Design review of the part built by this model. Coordinates are the model's own, in mm. A direction names the side the tool comes from. Round coordinates to 2 decimals unless told otherwise and drop trailing zeros. Write each loop counter-clockwise with the first axis right and the second up, starting at its lowest first coordinate (ties: lowest second). Pieces come first, ordered by that corner, then holes. Notation, with made-up numbers: (20.25, -19) -> (64.25, -19) arc R34 cw to (64.25, 16) -> close; hole circle Ø8 at (28.5, 87.5). An arc over 180 degrees is marked (long way). Write item = value, one per line. Start each with the question number.
Item 1: Add section C-C, the plane y = -11. State the section outline as (x, z) points.
Item 2: Machinability: for faces 1 (the flat face through (32, -20, 82)), 2 (the cylindrical face through (-304.222, -44.93, 73.268)), 3 (the flat face through (348.597, -20, 28)), which of the approach directions +Z, -Z, +X, -X, +Y, -Y give a long, thin tool a straight path to every point of the face, cutting with its end or side? Answer none if there is none.
Item 3: Add section B-B, the plane z = 125.5. State the section outline as (x, y) points, then the cut area to 3 significant figures.
Item 4: To check wall thickness, follow L1, parallel to Z at x = -25, y = -16.5; L2, parallel to Z at x = 13, y = -36; L3, parallel to X at y = -24, z = 125. State the ranges of each line that lie inside material, in increasing order.
Item 5: Add section D-D, the plane x = -129. State the section outline as (y, z) points.
Item 6: Add section A-A, the plane x = 25. State the section outline as (y, z) points.
Item 7: Mouldability with a two-part tool opening along Z and no side actions: class faces 4 (the cylindrical face through (-27.71, -19.72, 174.59)), 5 (the flat face through (-311, -50, 103)), 6 (the cylindrical face through (-290.5, -44.9, 75.8)) as released by +Z, released by -Z, zero draft, split by the parting line, or undercut.
from build123d import *

# Parameters (mm, degrees)
F1_W     = 560
F1_H     = 350
F1_W_2   = 111
F1_H_2   = 65
F1_R     = 68
F1_R_2   = 12.5
F1_W_3   = 64
F1_H_3   = 124
F1_W_4   = 30
F1_H_4   = 14
F1_R_3   = 11
F2_DEPTH = 40
F1_W_5   = 70
F3_DEPTH = 40
F4_DEPTH = 270
F6_DEPTH = 10


with BuildPart() as f2:
    # F1 (on Front) → F2 (new body)
    with BuildSketch(Plane.XZ):
        with Locations((-1.403241, 30.5)):
            Rectangle(F1_W, F1_H)
        with Locations((0, -22)):
            Rectangle(F1_W_2, F1_H_2, mode=Mode.SUBTRACT)
        with Locations((-180, 125.5)):
            Circle(F1_R, mode=Mode.SUBTRACT)
        with Locations((-25, 186.794207)):
            Circle(F1_R_2, mode=Mode.SUBTRACT)
        with Locations((0, 82.5)):
            Rectangle(F1_W_3, F1_H_3, mode=Mode.SUBTRACT)
        with Locations((0, 161.5)):
            Rectangle(F1_W_4, F1_H_4, mode=Mode.SUBTRACT)
        with Locations((25, 186.794207)):
            Circle(F1_R_3, mode=Mode.SUBTRACT)
        with Locations((180, 125.5)):
            Circle(F1_R, mode=Mode.SUBTRACT)
    extrude(amount=F2_DEPTH)

    # F1 (on Front) → F3 (join)
    with BuildSketch(Plane.XZ):
        with Locations((-316.403241, 30.5)):
            Rectangle(F1_W_5, F1_H)
        with Locations((313.596759, 30.5)):
            Rectangle(F1_W_5, F1_H)
    extrude(amount=F3_DEPTH)

    # F1 (on Front) → F4 (cut)
    with BuildSketch(Plane.XZ):
        with Locations((-180, 125.5)):
            Circle(F1_R)
        with Locations((180, 125.5)):
            Circle(F1_R)
        with Locations((-25, 186.794207)):
            Circle(F1_R_2)
        with Locations((25, 186.794207)):
            Circle(F1_R_3)
        with Locations((0, 161.5)):
            Rectangle(F1_W_4, F1_H_4)
        with Locations((0, 82.5)):
            Rectangle(F1_W_3, F1_H_3)
        with Locations((0, -22)):
            Rectangle(F1_W_2, F1_H_2)
    extrude(amount=-F4_DEPTH, mode=Mode.SUBTRACT)

    # F5 (on face) → F6 (join)
    with BuildSketch(Plane.XZ.offset(40)):
        with BuildLine():
            Line((-337.034283, 205.5), (-351.403241, 205.5))
            ThreePointArc((-351.403241, 205.5), (-302.927817, 71.70041), (-180, 0))
            ThreePointArc((-180, 0), (-291.71711, 77.380009), (-337.034283, 205.5))
        make_face()
    extrude(amount=F6_DEPTH)


solid = f2.part
Result set:
q1.outline = (-351.4, -144.5) -> (348.6, -144.5) -> (348.6, 205.5) -> (-351.4, 205.5) -> close; hole circle Ø136 at (-180, 125.5); hole (-55.5, -54.5) -> (55.5, -54.5) -> (55.5, 10.5) -> (-55.5, 10.5) -> close; hole circle Ø25 at (-25, 186.79); hole (-32, 20.5) -> (32, 20.5) -> (32, 144.5) -> (-32, 144.5) -> close; hole (-15, 154.5) -> (15, 154.5) -> (15, 168.5) -> (-15, 168.5) -> close; hole circle Ø22 at (25, 186.79); hole circle Ø136 at (180, 125.5)
q2.face_1 = +Y, -Y
q2.face_2 = -Z, -X, -Y
q2.face_3 = +Z, -Z, +X, +Y, -Y
q3.outline = (-351.4, -40) -> (-335.48, -40) -> (-335.48, -50) -> (-319.67, -50) -> (-319.67, -40) -> (-248, -40) -> (-248, 0) -> (-351.4, 0) -> close; (-112, -40) -> (-32, -40) -> (-32, 0) -> (-112, 0) -> close; (32, -40) -> (112, -40) -> (112, 0) -> (32, 0) -> close; (248, -40) -> (348.6, -40) -> (348.6, 0) -> (248, 0) -> close
q3.area = 14,700 mm²
q4.L1 = -144.5 to -54.5, 10.5 to 20.5, 144.5 to 174.29, 199.29 to 205.5
q4.L2 = -144.5 to -54.5, 10.5 to 20.5, 144.5 to 154.5, 168.5 to 205.5
q4.L3 = -351.4 to -248, -112 to -32, 32 to 112, 248 to 348.6
q5.outline = (-40, -144.5) -> (0, -144.5) -> (0, 80.52) -> (-40, 80.52) -> close; (-40, 170.48) -> (0, 170.48) -> (0, 205.5) -> (-40, 205.5) -> close
q6.outline = (-40, -144.5) -> (0, -144.5) -> (0, -54.5) -> (-40, -54.5) -> close; (-40, 10.5) -> (0, 10.5) -> (0, 20.5) -> (-40, 20.5) -> close; (-40, 144.5) -> (0, 144.5) -> (0, 175.79) -> (-40, 175.79) -> close; (-40, 197.79) -> (0, 197.79) -> (0, 205.5) -> (-40, 205.5) -> close
q7.face_4 = undercut
q7.face_5 = zero draft
q7.face_6 = released by +Z
